Autodesk Inventor part; units mm, degrees
ref_plane "YZ Plane" through (0, 0, 0) normal (1, 0, 0) x (0, 1, 0)
ref_plane "XZ Plane" through (0, 0, 0) normal (0, 1, 0) x (-1, 0, 0)
ref_plane "XY Plane" through (0, 0, 0) normal (0, 0, 1) x (1, 0, 0)
sketch "Sketch1" plane through (0, 0, 0) normal (0, 0, 1) x (1, 0, 0)
  line L0 (-3.6, 4.2059) -> (-3.6, -4.2059)
  line L1 (-3.6, -4.2059) -> (-2.3111, -6.0753)
  arc A0 (-2.3111, -6.0753) -> (0, -6.5) centre (0, 0) ccw
  line L2 (0, -6.5) -> (10, -6.5)
  line L3 (10, -6.5) -> (10, 6.5)
  line L4 (10, 6.5) -> (0, 6.5)
  arc A1 (0, 6.5) -> (-2.3111, 6.0753) centre (0, 0) ccw
  line L5 (-2.3111, 6.0753) -> (-3.6, 4.2059)
  circle A2 centre (0, 0) radius 2.6
extrude "Extrusion1" add sketch "Sketch1" against normal blind 0.9906
sketch "Sketch2" plane through (0, 0, 0) normal (0, 0, 1) x (1, 0, 0)
  line L0 (-1.0714, 3.7) -> (1.0714, 3.7)
  line L1 (-1.0714, 3.4) -> (-1.0714, 3.7)
  line L2 (1.0714, 3.4) -> (-1.0714, 3.4)
  line L3 (1.0714, 3.7) -> (1.0714, 3.4)
  line L4 (-1.0714, -3.4) -> (1.0714, -3.4)
  line L5 (-1.0714, -3.7) -> (-1.0714, -3.4)
  line L6 (1.0714, -3.7) -> (-1.0714, -3.7)
  line L7 (1.0714, -3.4) -> (1.0714, -3.7)
extrude "Extrusion2" cut sketch "Sketch2" against normal up to next
properties part number "276-2181-012 Rev1" material "Steel"
Verification items for the finished model (mm, model axes). A direction names the side the tool comes from. Give positions to 0.01 mm unless a question says otherwise; leave off trailing zeros. Write each loop counter-clockwise with the first axis right and the second up, starting at its lowest first coordinate (ties: lowest second). Pieces come first, ordered by that corner, then holes. Notation, with made-up numbers: (-2, 63) - (20, 63) arc R15 ccw to (20, 89) - close; hole circle Ø2 at (5.5, -12.5). An arc over 180 degrees is marked (long way). Answer as CSV lines item,"result". Start each with the question number.
1. Draft check along Y on faces 3 (the face through (0, -3.4, -0.5)), 4 (the face through (-1.19, -6.39, -0.49)), 5 (the face through (5.1, 6.5, -0.5)), 6 (the face through (10, -0.1, -0.5)). Enter one of: pulls with the +Y half, pulls with the -Y half, needs draft (parallel to the pull), parting line crosses it, or undercut.
2. Depth check by flat-ended pin: pin 1 (5 mm diameter, centred on x = -0.5, y = 1, fed in from -Z). Enter the tip coordinate at first touch or a pass-through.
3. Thickness scan on line 1 (Y direction, x = 0, z = -0.45); line 2 (X direction, y = 4.5, z = -0.05); line 3 (X direction, y = 4.75, z = -0.55). Record the ranges inside material, lowest first.
4. Sectioned sample at C-C (y = -1.5). Record the boundary of the cut face in (x, z).
5. Sectioned sample at B-B (y = 1). Record the boundary of the cut face in (x, z), then the cut area to 3 significant figures.
6. Set-up check for faces 1 (the face through (3, 0, -0.991)), 2 (the face through (0, 3.7, -0.5)): record each of +Z, -Z, +X, -X, +Y, -Y from which the full face is reachable in a straight line by a thin tool's end or side.
7. Sectioned sample at D-D (y = -5.25). Record the boundary of the cut face in (x, z), then the cut area to 3 significant figures.
8. Sectioned sample at A-A (z = -0.3). Record the boundary of the cut face in (x, y), then the cut area to 3 significant figures.
Derived:
1,face 3,"undercut"
1,face 4,"pulls with the -Y half"
1,face 5,"pulls with the +Y half"
1,face 6,"needs draft"
2,pin 1,"z = -0.99"
3,line 1,"-6.5 to -3.7, -3.4 to -2.6, 2.6 to 3.4, 3.7 to 6.5"
3,line 2,"-3.4 to 10"
3,line 3,"-3.22 to 10"
4,outline,"(-3.6, -0.99) - (-2.12, -0.99) - (-2.12, 0) - (-3.6, 0) - close; (2.12, -0.99) - (10, -0.99) - (10, 0) - (2.12, 0) - close"
5,outline,"(-3.6, -0.99) - (-2.4, -0.99) - (-2.4, 0) - (-3.6, 0) - close; (2.4, -0.99) - (10, -0.99) - (10, 0) - (2.4, 0) - close"
5,area,"8.72 mm²"
6,face 1,"-Z, +X, -X, +Y, -Y"
6,face 2,"+Z, -Z"
7,outline,"(-2.88, -0.99) - (10, -0.99) - (10, 0) - (-2.88, 0) - close"
7,area,"12.8 mm²"
8,outline,"(-3.6, -4.21) - (-2.31, -6.08) arc R6.5 ccw to (0, -6.5) - (10, -6.5) - (10, 6.5) - (0, 6.5) arc R6.5 ccw to (-2.31, 6.08) - (-3.6, 4.21) - close; hole circle Ø5.2 at (0, 0); hole (-1.07, -3.7) - (1.07, -3.7) - (1.07, -3.4) - (-1.07, -3.4) - close; hole (-1.07, 3.4) - (1.07, 3.4) - (1.07, 3.7) - (-1.07, 3.7) - close"
8,area,"150 mm²"
